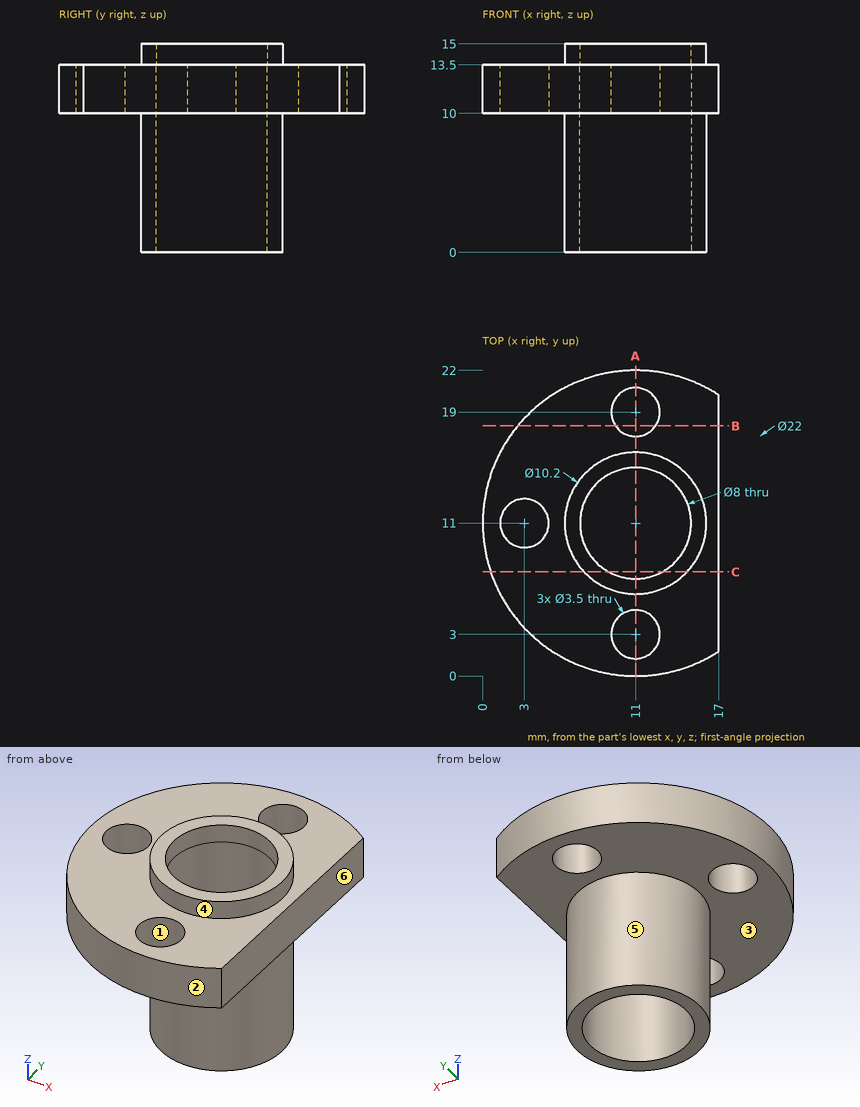
The figure shows three views and two pictorial views of one solid part (mm, origin at its lowest corner). Answer the questions. A direction names the side the tool comes from. Give positions to 0.01 mm unless a question says otherwise; leave off trailing zeros. Order: outer loops, then holes, each group sorted by start corner. A loop starts at its lowest first (then second) coordinate and runs counter-clockwise, first axis right, second up. Notation, with made-up numbers: (57.5, -34.5) -> (111.5, -34.5) arc R24 cw to (111.5, -24.5) -> close; hole circle Ø5 at (51.5, 14.25). An arc over 180 degrees is marked (long way). One line per item, written item: value.
1) Find section B-B, the plane y = 18. Determine the outline of the cut face in (x, z).
Reported:
outline: (2.51, 10) -> (9.56, 10) -> (9.56, 13.5) -> (2.51, 13.5) -> close; (12.44, 10) -> (17, 10) -> (17, 13.5) -> (12.44, 13.5) -> close
2) Flat-ended cylindrical pins translate along their axes: P1, Ø6, axis at x = 2.5, y = 4.5, coming from the +Z side; P2, Ø5.5, axis at x = 11, y = 19, coming from the -Z side. Find the tip coordinate at first contact, or state that the pin passes through.
Reported:
P1: stops at z = 13.5
P2: stops at z = 10
3) Find section C-C, the plane y = 7.5. Determine the outline of the cut face in (x, z).
Reported:
outline: (0.57, 10) -> (7.29, 10) -> (7.29, 0) -> (9.06, 0) -> (9.06, 15) -> (7.29, 15) -> (7.29, 13.5) -> (0.57, 13.5) -> close; (12.94, 0) -> (14.71, 0) -> (14.71, 10) -> (17, 10) -> (17, 13.5) -> (14.71, 13.5) -> (14.71, 15) -> (12.94, 15) -> close
4) Find the intervals of material crossed by line 1 (Y direction, x = 11, z = 11.9); line 2 (Y direction, x = 11, z = 8.5); line 3 (X direction, y = 11.25, z = 13.25), in increasing order.
Reported:
line 1: y = 0 to 1.25, 4.75 to 7, 15 to 17.25, 20.75 to 22
line 2: y = 5.9 to 7, 15 to 16.1
line 3: x = 0 to 1.27, 4.73 to 7.01, 14.99 to 17
5) A tool of negligible diameter and unlimited length cuts with its end or side. For the marked faces 4, 5 and 6, from which of +Z, -Z, +X, -X, +Y, -Y can it reach the whole face along a straight path? Write none if from no direction.
Reported:
face 4: +Z
face 5: -Z
face 6: +Z, -Z, +X, +Y, -Y
6) Determine the mould class of the marked faces 1, 2 and 3 for opening direction Y: pulls with the +Y half, pulls with the -Y half, needs draft (parallel to the pull), parting line crosses it, or undercut.
Reported:
face 1: undercut
face 2: parting line crosses it
face 3: needs draft
7) Find section A-A, the plane x = 11. Determine the outline of the cut face in (y, z).
Reported:
outline: (0, 10) -> (1.25, 10) -> (1.25, 13.5) -> (0, 13.5) -> close; (4.75, 10) -> (5.9, 10) -> (5.9, 0) -> (7, 0) -> (7, 15) -> (5.9, 15) -> (5.9, 13.5) -> (4.75, 13.5) -> close; (15, 0) -> (16.1, 0) -> (16.1, 10) -> (17.25, 10) -> (17.25, 13.5) -> (16.1, 13.5) -> (16.1, 15) -> (15, 15) -> close; (20.75, 10) -> (22, 10) -> (22, 13.5) -> (20.75, 13.5) -> close
